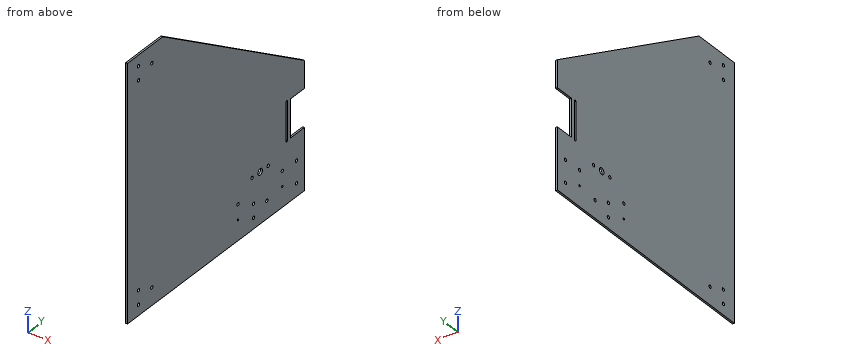
```python
from build123d import *

# Parameters (mm, degrees)
SKETCH1_R                  = 2.5
SKETCH1_R_2                = 5
BOSS_EXTRUDE1_DEPTH        = 5
CONVERT_SOLID1_OUTLINE_R   = 2.5
CONVERT_SOLID1_OUTLINE_R_2 = 5
CONVERT_SOLID1_DEPTH       = 2
SKETCH6_R                  = 2.5
CUT_EXTRUDE1_DEPTH         = 10
SKETCH7_R                  = 2.5
CUT_EXTRUDE2_DEPTH         = 10
SKETCH8_R                  = 2.5
CUT_EXTRUDE3_DEPTH         = 10
SKETCH9_R                  = 1.5
CUT_EXTRUDE4_DEPTH         = 10
SKETCH10_W                 = 60
SKETCH10_H                 = 32
CUT_EXTRUDE5_DEPTH         = 10


# Read off the part's stored shape, not the designer's step: Convert-Solid1
with BuildPart() as part:
    # Sketch1 → Boss-Extrude1 (new body)
    with BuildSketch(Plane(origin=(0, 0, 0), x_dir=(0, 0, -1), z_dir=(1, 0, 0))):
        Polygon((0, 0), (400, 0), (400, 400), (200, 400), (0, 80), align=None)
        with Locations((344, 350)):
            Circle(SKETCH1_R, mode=Mode.SUBTRACT)
        with Locations((344, 250)):
            Circle(SKETCH1_R, mode=Mode.SUBTRACT)
        with Locations((320, 300)):
            Circle(SKETCH1_R_2, mode=Mode.SUBTRACT)
        with Locations((320, 318.25)):
            Circle(SKETCH1_R, mode=Mode.SUBTRACT)
        with Locations(Location((320, 281.75, 0), (0, 0, 180))):
            Circle(SKETCH1_R, mode=Mode.SUBTRACT)
    extrude(amount=BOSS_EXTRUDE1_DEPTH)

    # Convert-Solid1 outline → Convert-Solid1 (cut)
    with BuildSketch(Plane.YZ):
        Polygon((80, 0), (0, 0), (0, -400), (400, -400), (400, -200), align=None)
        with Locations((250, -344)):
            Circle(CONVERT_SOLID1_OUTLINE_R, mode=Mode.SUBTRACT)
        with Locations((281.75, -320)):
            Circle(CONVERT_SOLID1_OUTLINE_R, mode=Mode.SUBTRACT)
        with Locations((300, -320)):
            Circle(CONVERT_SOLID1_OUTLINE_R_2, mode=Mode.SUBTRACT)
        with Locations((350, -344)):
            Circle(CONVERT_SOLID1_OUTLINE_R, mode=Mode.SUBTRACT)
        with Locations((318.25, -320)):
            Circle(CONVERT_SOLID1_OUTLINE_R, mode=Mode.SUBTRACT)
    extrude(amount=CONVERT_SOLID1_DEPTH, mode=Mode.SUBTRACT)

    # Sketch6 → Cut-Extrude1 (cut)
    with BuildSketch(Plane(origin=(5, 0, 0), x_dir=(0, 0, -1), z_dir=(1, 0, 0))):
        with Locations((28, 55)):
            Circle(SKETCH6_R)
        with Locations((39, 25)):
            Circle(SKETCH6_R)
        with Locations(Location((17, 25, 0), (0, 0, 180))):
            Circle(SKETCH6_R)
        with Locations((383, 25)):
            Circle(SKETCH6_R)
        with Locations(Location((361, 25, 0), (0, 0, 180))):
            Circle(SKETCH6_R)
        with Locations(Location((372, 55, 0), (0, 0, 180))):
            Circle(SKETCH6_R)
    extrude(amount=-CUT_EXTRUDE1_DEPTH, mode=Mode.SUBTRACT)

    # Sketch7 → Cut-Extrude2 (cut)
    with BuildSketch(Plane.ZY.offset(-2)):
        with Locations((-372, 315)):
            Circle(SKETCH7_R)
        with Locations((-361, 285)):
            Circle(SKETCH7_R)
        with Locations(Location((-383, 285, 0), (0, 0, 180))):
            Circle(SKETCH7_R)
    extrude(amount=-CUT_EXTRUDE2_DEPTH, mode=Mode.SUBTRACT)

    # Sketch8 → Cut-Extrude3 (cut)
    with BuildSketch(Plane.ZY.offset(-2)):
        with Locations((-344.5, 382)):
            Circle(SKETCH8_R)
        with Locations((-379.5, 382)):
            Circle(SKETCH8_R)
    extrude(amount=-CUT_EXTRUDE3_DEPTH, mode=Mode.SUBTRACT)

    # Sketch9 → Cut-Extrude4 (cut)
    with BuildSketch(Plane.ZY.offset(-2)):
        with Locations((-368, 350)):
            Circle(SKETCH9_R)
        with Locations((-368, 250)):
            Circle(SKETCH9_R)
    extrude(amount=-CUT_EXTRUDE4_DEPTH, mode=Mode.SUBTRACT)

    # Sketch10 → Cut-Extrude5 (cut)
    with BuildSketch(Plane(origin=(5, 0, 0), x_dir=(0, 0, -1), z_dir=(1, 0, 0))):
        with Locations((273, 384)):
            Rectangle(SKETCH10_W, SKETCH10_H)
        with BuildLine():
            Line((243, 361.5), (303, 361.5))
            ThreePointArc((303, 361.5), (304.5, 360), (303, 358.5))
            Line((303, 358.5), (243, 358.5))
            ThreePointArc((243, 358.5), (241.5, 360), (243, 361.5))
        make_face()
    extrude(amount=-CUT_EXTRUDE5_DEPTH, mode=Mode.SUBTRACT)


solid = part.part
```
Could you check a few things on this model? Use its own coordinates, in mm. Coordinates: 2 decimals unless noted, no trailing zeros. Write each loop counter-clockwise with the first axis right and the second up, starting at its lowest first coordinate (ties: lowest second). Pieces come first, ordered by that corner, then holes. Notation, with made-up numbers: (88, 81.5) -> (141, 81.5) arc R27 cw to (141, 97.5) -> close; hole circle Ø2 at (48, 44.25). An arc over 180 degrees is marked (long way). One line per question, with ' | ' between items. Start each with the question number.
1. Please list where these lines run through material, in increasing order: line 1 along Y through (x, z) = (3.05, -344.5); line 2 along Y through (x, z) = (3.95, -320); line 3 along Z through (x, y) = (3.55, 285) (3 decimals).
2. If we section it at C-C (y = 332): Please give me the cut outline in (x, z).
3. If we section it at B-B (z = -133.5): Please give me the cut outline in (x, y), and give its area (3 significant figures).
4. Will these pins go through, and if not, where does the flat tip stop? P1, Ø3, axis at y = 25, z = -39, coming from the +X side; P2, Ø1.5, axis at x = 3.5, z = -43.5, coming from the +Y side; P3, Ø3.5, axis at y = 350, z = -368, coming from the -X side.
5. If we section it at A-A (x = 3.85): Count the separate pieces of the cut face and the enclosed holes in it, and give its area (3 significant figures).
Return value:
1) line 1: y = 0 to 247.55, 252.45 to 347.55, 352.45 to 379.5, 384.5 to 400 | line 2: y = 0 to 279.25, 284.25 to 295, 305 to 315.75, 320.75 to 400 | line 3: z = -400 to -385.5, -380.5 to -363.5, -358.5 to -128.125
2) outline: (2, -400) -> (5, -400) -> (5, -157.5) -> (2, -157.5) -> close
3) outline: (2, 0) -> (5, 0) -> (5, 293.6) -> (2, 293.6) -> close | area: 881 mm²
4) P1: passes through | P2: stops at y = 150.8 | P3: stops at x = 2
5) separate pieces: 1 | enclosed holes: 19 | area: 126,000 mm²
